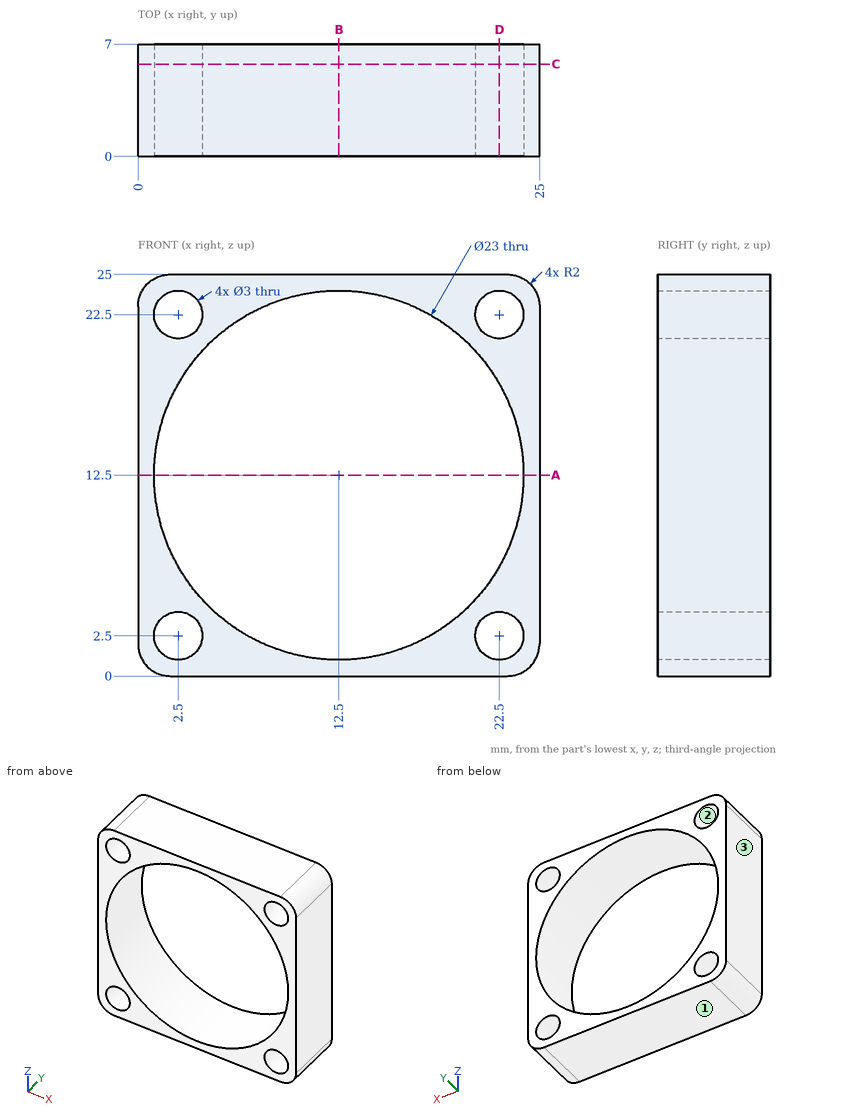
Could you check a few things on this drawing? It's one solid part, dimensions in mm from its lowest x, y, z. Round coordinates to 2 decimals unless told otherwise and drop trailing zeros. Order: outer loops, then holes, each group sorted by start corner. A loop starts at its lowest first (then second) coordinate and runs counter-clockwise, first axis right, second up.
(1) Imagine slicing it at B-B (x = 12.5). Write out the boundary of the cut face in (y, z), plus the area to 3 significant figures.
Response values:
outline: (0, 0) - (7, 0) - (7, 1) - (0, 1) - close; (0, 24) - (7, 24) - (7, 25) - (0, 25) - close
area: 14.0 mm2
(2) Imagine slicing it at A-A (z = 12.5). Write out the boundary of the cut face in (x, y), plus the area to 3 significant figures.
Response values:
outline: (0, 0) - (1, 0) - (1, 7) - (0, 7) - close; (24, 0) - (25, 0) - (25, 7) - (24, 7) - close
area: 14.0 mm2
(3) Imagine slicing it at C-C (y = 5.75). Write out the boundary of the cut face in (x, z).
Response values:
outline: (0, 2) arc R2 ccw to (2, 0) - (23, 0) arc R2 ccw to (25, 2) - (25, 23) arc R2 ccw to (23, 25) - (2, 25) arc R2 ccw to (0, 23) - close; hole circle Ø3 at (2.5, 2.5); hole circle Ø23 at (12.5, 12.5); hole circle Ø3 at (2.5, 22.5); hole circle Ø3 at (22.5, 2.5); hole circle Ø3 at (22.5, 22.5)
(4) Imagine slicing it at D-D (x = 22.5). Write out the boundary of the cut face in (y, z).
Response values:
outline: (0, 0) - (7, 0) - (7, 1) - (0, 1) - close; (0, 4) - (7, 4) - (7, 6.82) - (0, 6.82) - close; (0, 18.18) - (7, 18.18) - (7, 21) - (0, 21) - close; (0, 24) - (7, 24) - (7, 25) - (0, 25) - close
(5) I'm going to push flat-ended pins straight in: pin 1 (2.5 mm diameter, centred on x = 2.5, z = 2.5, fed in from +Y); pin 2 (4 mm diameter, centred on x = 2.5, z = 22.5, fed in from +Y). Where does each tip first touch, or does it pass through?
Response values:
pin 1: passes through
pin 2: stops at y = 7
(6) If we mould it in two halves opening along X, with no side actions, what happens to the marked faces 1, 2 and 3? For each: released by +X, released by -X, zero draft, split by the parting line, or undercut.
Response values:
face 1: zero draft
face 2: undercut
face 3: released by -X
(7) Please list where these lines run through material, in increasing order: line 1 along Z through (x, y) = (3.25, 2); line 2 along Z through (x, y) = (4.75, 2); line 3 along X through (y, z) = (5.25, 22.5).
Response values:
line 1: z = 0 to 1.2, 3.8 to 5.67, 19.33 to 21.2, 23.8 to 25
line 2: z = 0 to 4, 21 to 25
line 3: x = 0 to 1, 4 to 6.82, 18.18 to 21, 24 to 25
